```python
from build123d import *

# Parameters (mm, degrees)
SKETCH_1_R          = 13
EXTRUDE_1_DEPTH     = 7
SKETCH_6_R          = 14
EXTRUDE_4_DEPTH     = 7
SKETCH_2_R          = 12
CUT_EXTRUDE_1_DEPTH = 3
CUT_EXTRUDE_2_DEPTH = 22


with BuildPart() as part:
    # 草图1 → 凸台-拉伸1 (new body)
    with BuildSketch(Plane(origin=(0, 0, 0), x_dir=(1, 0, 0), z_dir=(0, 1, 0))):
        with Locations(Location((0, 0, 0), (0, 0, 270))):
            Circle(SKETCH_1_R)
    extrude(amount=EXTRUDE_1_DEPTH)

    # 草图6 → 凸台-拉伸4 (add, through all)
    with BuildSketch(Plane(origin=(0, 7, 0), x_dir=(1, 0, 0), z_dir=(0, 1, 0))):
        with Locations(Location((0, 0, 0), (0, 0, 270))):
            Circle(SKETCH_6_R)
    extrude(amount=-EXTRUDE_4_DEPTH)

    # 草图2 → 切除-拉伸1 (cut)
    with BuildSketch(Plane(origin=(0, 7, 0), x_dir=(1, 0, 0), z_dir=(0, 1, 0))):
        with Locations(Location((0, 0, 0), (0, 0, 270))):
            Circle(SKETCH_2_R)
    extrude(amount=-CUT_EXTRUDE_1_DEPTH, mode=Mode.SUBTRACT)

    # 草图7 → 切除-拉伸2 (cut, through all)
    with BuildSketch(Plane(origin=(0, 7, 0), x_dir=(1, 0, 0), z_dir=(0, 1, 0))):
        Polygon((-15.646830527, 4.142221687), (-12.567085782, 3.326913727), (-12.296421758, 4.349320163), (-15.376166503, 5.164628122), align=None)
        Polygon((-14.689830765, 6.79633564), (-11.798451005, 5.458621977), (-11.354359961, 6.418495447), (-14.245739722, 7.756209109), align=None)
        Polygon((-13.28648793, 9.243946373), (-10.671326264, 7.42447276), (-10.067301683, 8.292647994), (-12.682463348, 10.112121607), align=None)
        Polygon((-11.479441881, 11.410684473), (-9.219958675, 9.164734695), (-8.474353537, 9.914832629), (-10.733836743, 12.160782407), align=None)
        Polygon((-9.3235988, 13.230714699), (-7.488447307, 10.626530804), (-6.623916447, 11.235760092), (-8.45906794, 13.839943987), align=None)
        Polygon((-6.884462888, 14.648736355), (-5.529403257, 11.765445152), (-4.572215008, 12.215294669), (-5.927274639, 15.098585872), align=None)
        Polygon((-4.236146054, 15.621663569), (-3.402351087, 12.546872402), (-2.381589129, 12.8236737), (-3.215384096, 15.898464866), align=None)
        Polygon((-1.459116066, 16.11993444), (-1.171920201, 12.947069284), (-0.11859987, 13.042411894), (-0.405795735, 16.21527705), align=None)
        Polygon((1.362248425, 16.12840926), (1.094118888, 12.953876017), (2.147992986, 12.864863002), (2.416122524, 16.039396246), align=None)
        Polygon((4.142221687, 15.646830527), (3.326913727, 12.567085782), (4.349320163, 12.296421758), (5.164628122, 15.376166503), align=None)
        Polygon((6.79633564, 14.689830765), (5.458621977, 11.798451005), (6.418495447, 11.354359961), (7.756209109, 14.245739722), align=None)
        Polygon((9.243946373, 13.28648793), (7.42447276, 10.671326264), (8.292647994, 10.067301683), (10.112121607, 12.682463348), align=None)
        Polygon((11.410684473, 11.479441881), (9.164734695, 9.219958675), (9.914832629, 8.474353537), (12.160782407, 10.733836743), align=None)
        Polygon((13.230714699, 9.3235988), (10.626530804, 7.488447307), (11.235760092, 6.623916447), (13.839943987, 8.45906794), align=None)
        Polygon((14.648736355, 6.884462888), (11.765445152, 5.529403257), (12.215294669, 4.572215008), (15.098585872, 5.927274639), align=None)
        Polygon((15.621663569, 4.236146054), (12.546872402, 3.402351087), (12.8236737, 2.381589129), (15.898464866, 3.215384096), align=None)
        Polygon((16.11993444, 1.459116066), (12.947069284, 1.171920201), (13.042411894, 0.11859987), (16.21527705, 0.405795735), align=None)
        Polygon((16.12840926, -1.362248425), (12.953876017, -1.094118888), (12.864863002, -2.147992986), (16.039396246, -2.416122524), align=None)
        Polygon((15.646830527, -4.142221687), (12.567085782, -3.326913727), (12.296421758, -4.349320163), (15.376166503, -5.164628122), align=None)
        Polygon((14.689830765, -6.79633564), (11.798451005, -5.458621977), (11.354359961, -6.418495447), (14.245739722, -7.756209109), align=None)
        Polygon((13.28648793, -9.243946373), (10.671326264, -7.42447276), (10.067301683, -8.292647994), (12.682463348, -10.112121607), align=None)
        Polygon((11.479441881, -11.410684473), (9.219958675, -9.164734695), (8.474353537, -9.914832629), (10.733836743, -12.160782407), align=None)
        Polygon((9.3235988, -13.230714699), (7.488447307, -10.626530804), (6.623916447, -11.235760092), (8.45906794, -13.839943987), align=None)
        Polygon((6.884462888, -14.648736355), (5.529403257, -11.765445152), (4.572215008, -12.215294669), (5.927274639, -15.098585872), align=None)
        Polygon((4.236146054, -15.621663569), (3.402351087, -12.546872402), (2.381589129, -12.8236737), (3.215384096, -15.898464866), align=None)
        Polygon((1.459116066, -16.11993444), (1.171920201, -12.947069284), (0.11859987, -13.042411894), (0.405795735, -16.21527705), align=None)
        Polygon((-1.362248425, -16.12840926), (-1.094118888, -12.953876017), (-2.147992986, -12.864863002), (-2.416122524, -16.039396246), align=None)
        Polygon((-4.142221687, -15.646830527), (-3.326913727, -12.567085782), (-4.349320163, -12.296421758), (-5.164628122, -15.376166503), align=None)
        Polygon((-6.79633564, -14.689830765), (-5.458621977, -11.798451005), (-6.418495447, -11.354359961), (-7.756209109, -14.245739722), align=None)
        Polygon((-9.243946373, -13.28648793), (-7.42447276, -10.671326264), (-8.292647994, -10.067301683), (-10.112121607, -12.682463348), align=None)
        Polygon((-11.410684473, -11.479441881), (-9.164734695, -9.219958675), (-9.914832629, -8.474353537), (-12.160782407, -10.733836743), align=None)
        Polygon((-13.230714699, -9.3235988), (-10.626530804, -7.488447307), (-11.235760092, -6.623916447), (-13.839943987, -8.45906794), align=None)
        Polygon((-14.648736355, -6.884462888), (-11.765445152, -5.529403257), (-12.215294669, -4.572215008), (-15.098585872, -5.927274639), align=None)
        Polygon((-15.621663569, -4.236146054), (-12.546872402, -3.402351087), (-12.8236737, -2.381589129), (-15.898464866, -3.215384096), align=None)
        Polygon((-16.11993444, -1.459116066), (-12.947069284, -1.171920201), (-13.042411894, -0.11859987), (-16.21527705, -0.405795735), align=None)
        Polygon((-16.12840926, 1.362248425), (-12.953876017, 1.094118888), (-12.864863002, 2.147992986), (-16.039396246, 2.416122524), align=None)
    extrude(amount=-CUT_EXTRUDE_2_DEPTH, mode=Mode.SUBTRACT)


solid = part.part
```
Geometry: final body of the model. Coordinates: model frame, mm. A direction names the side the tool comes from. Give positions to 0.01 mm unless a question says otherwise; leave off trailing zeros. Use CSV: the item, a comma, the result in double quotes.
(1) Pull-direction query (X, two-part tool) for faces 4 (the face through (10.4, 3.55, 9.37)), 5 (the face through (-13.34, 3.55, -2.19)), 6 (the face through (-7.1, 3.5, -10.9)); classes: released by +X, released by -X, zero draft, split by the parting line, or undercut.
From the geometry:
face 4,"released by +X"
face 5,"released by -X"
face 6,"undercut"
(2) Access query for faces 1 (the face through (3.604, 5.521, 11.446)), 2 (the face through (12.683, 3.549, -2.899)), 3 (the face through (-2.19, 3.55, 13.34)). Directions: +Z, -Z, +X, -X, +Y, -Y. A direction counts if a zero-diameter tool reaches every point of the face in a straight line with its end or side. Return the directions, or none.
From the geometry:
face 1,"+Y"
face 2,"+Y, -Y"
face 3,"+Z, +Y, -Y"
(3) First-contact query: P1, Ø1, axis at y = 2.5, z = 5.5, coming from the +X side; P2, Ø2, axis at x = 4, y = 6, coming from the +Z side; P3, Ø12, axis at x = -2, z = 2, coming from the +Y side. Flat tips, straight axial feed; report the tip coordinate or a pass-through.
From the geometry:
P1,"x = 13.08"
P2,"z = 13.51"
P3,"y = 4"
(4) Ray query, line 1 along X through (y, z) = (5.7, 0); line 2 along Z through (x, y) = (-10.75, 6.5); line 3 along X through (y, z) = (1.5, -10.75). Return the intervals inside material, ascending. Write a range as [from, to].
From the geometry:
line 1,"[-14, -12], [12, 14]"
line 2,"[-8.97, -8.77], [-7.48, -5.33], [5.33, 7.31], [7.58, 8.97]"
line 3,"[-8.97, -7.58], [-7.31, 7.48], [8.77, 8.97]"
